from build123d import *

# Parameters (mm, degrees)
SKETCH1_W           = 25
SKETCH1_H           = 7.15
BOSS_EXTRUDE1_DEPTH = 12
BOSS_EXTRUDE2_DEPTH = 3
CUT_EXTRUDE1_DEPTH  = 21
SKETCH4_R           = 9
CUT_EXTRUDE2_DEPTH  = 10
CHAMFER1_SIZE       = 5
CHAMFER1_SIZE2      = 20
CHAMFER2_SIZE       = 5
SKETCH6_R           = 1.05
CUT_EXTRUDE3_DEPTH  = 10
CUT_EXTRUDE4_DEPTH  = 4.5
FILLET1_R           = 3
FILLET2_R           = 1.5


with BuildPart() as part:
    # Sketch1 → Boss-Extrude1 (new body)
    with BuildSketch(Plane.XY):
        with Locations((12.5, 3.575)):
            Rectangle(SKETCH1_W, SKETCH1_H)
    extrude(amount=BOSS_EXTRUDE1_DEPTH)

    # Sketch2 → Boss-Extrude2 (add)
    with BuildSketch(Plane(origin=(0, 7.15, 0), x_dir=(1, 0, 0), z_dir=(0, 1, 0))):
        with BuildLine():
            Line((15, -12), (15, -6))
            Line((15, -6), (15, 0))
            Line((15, 0), (-5.804949202, 4.737516245))
            ThreePointArc((-5.804949202, 4.737516245), (-19.262380692, -6), (-5.804949202, -16.737516245))
            Line((-5.804949202, -16.737516245), (15, -12))
        make_face()
    extrude(amount=-BOSS_EXTRUDE2_DEPTH)

    # Sketch3 → Cut-Extrude1 (cut)
    with BuildSketch(Plane.XZ.offset(-4.15)):
        Polygon((2.25, 6), (2.25, 12), (0, 12), (0, 0), (2.25, 0), align=None)
    extrude(amount=CUT_EXTRUDE1_DEPTH, mode=Mode.SUBTRACT)

    # Sketch4 → Cut-Extrude2 (cut)
    with BuildSketch(Plane.XZ.offset(-4.15)):
        with Locations(Location((-8.25, 6, 0), (0, 0, 270))):
            Circle(SKETCH4_R)
    extrude(amount=-CUT_EXTRUDE2_DEPTH, mode=Mode.SUBTRACT)

    # Chamfer1
    chamfer1_edges = [part.edges().sort_by_distance(p)[0] for p in [
        (25, 7.15, 6),
    ]]
    chamfer1_side = [part.faces().sort_by_distance(p)[0] for p in [
        (25, 3.575, 6),
    ]]
    chamfer(chamfer1_edges, length=CHAMFER1_SIZE, length2=CHAMFER1_SIZE2, reference=chamfer1_side[0])

    # Chamfer2
    chamfer2_edges = [part.edges().sort_by_distance(p)[0] for p in [
        (25, 1.075, 0),
        (25, 1.075, 12),
    ]]
    chamfer(chamfer2_edges, length=CHAMFER2_SIZE)

    # Sketch6 → Cut-Extrude3 (cut)
    with BuildSketch(Plane(origin=(0, 7.15, 0), x_dir=(1, 0, 0), z_dir=(0, 1, 0))):
        with Locations(Location((7.829893366, -6, 0), (0, 0, 180))):
            Circle(SKETCH6_R)
        with Locations(Location((17.829893366, -6, 0), (0, 0, 180))):
            Circle(SKETCH6_R)
    extrude(amount=-CUT_EXTRUDE3_DEPTH, mode=Mode.SUBTRACT)

    # Sketch7 → Cut-Extrude4 (cut)
    with BuildSketch(Plane(origin=(0, 7.15, 0), x_dir=(1, 0, 0), z_dir=(0, 1, 0))):
        with BuildLine():
            Line((7.829893366, -2), (17.829893366, -2))
            ThreePointArc((17.829893366, -2), (21.829893366, -6), (17.829893366, -10))
            Line((17.829893366, -10), (7.829893366, -10))
            ThreePointArc((7.829893366, -10), (3.829893366, -6), (7.829893366, -2))
        make_face()
    extrude(amount=-CUT_EXTRUDE4_DEPTH, mode=Mode.SUBTRACT)

    # Fillet1
    fillet1_edges = [part.edges().sort_by_distance(p)[0] for p in [
        (2.25, 2.075, 0),
        (2.25, 2.075, 12),
    ]]
    fillet(fillet1_edges, radius=FILLET1_R)

    # Fillet2
    fillet2_edges = [part.edges().sort_by_distance(p)[0] for p in [
        (10.125, 4.15, 0),
        (3.128679656, 4.15, 0.878679656),
        (2.25, 4.15, 6),
        (3.128679656, 4.15, 11.121320344),
        (10.125, 4.15, 12),
    ]]
    fillet(fillet2_edges, radius=FILLET2_R)


solid = part.part
Model file for the job. Use its own axes, mm. A direction names the side the tool comes from. Round coordinates to 2 decimals unless told otherwise and drop trailing zeros. Order: outer loops, then holes, each group sorted by start corner. A loop starts at its lowest first (then second) coordinate and runs counter-clockwise, first axis right, second up.
(1) Pull direction X, two halves, no side cores. Call faces 1 (the face through (6.83, 1.34, 6.32)), 2 (the face through (13, 2, 12)), 3 (the face through (13.472, 5.032, 1.67)): released by +X, released by -X, zero draft, split by the parting line, or undercut.
(2) Band-saw the part on B-B (y = 1). List the corners of the cut face in (x, z), then the cut area to 3 significant figures.
(3) Band-saw the part on C-C (z = 5.5). Give the number of separate pieces and of enclosed holes in the cut face, then the cut area to 3 significant figures.
(4) 3-axis set-ups, long thin cutter, end or side, ignore diameter. For faces 4 (the face through (3.15, 1.31, 11.14)), 5 (the face through (3.15, 1.31, 0.86)), 6 (the face through (3.83, 4.93, 6.09)): which of +Z, -Z, +X, -X, +Y, -Y reach the whole face in a straight line?
(5) Pin check, flat tips, straight feed: pin 1 (3 mm diameter, centred on x = 14.5, y = 4, fed in from +Z); pin 2 (11 mm diameter, centred on x = -4.5, z = 6.5, fed in from -Y); pin 3 (3 mm diameter, centred on x = 11.5, y = 5, fed in from -Z); pin 4 (1.9 mm diameter, centred on x = 7.83, z = 6, fed in from -Y). Stop position of each tip, or through.
(6) Band-saw the part on D-D (x = 16). List the corners of the cut face in (y, z).
(7) Band-saw the part on A-A (x = -8.25). List the corners of the cut face in (y, z).
(8) Drill centre lines: line 1 (X direction, y = 6.15, z = 6); line 2 (Y direction, x = -5, z = 14.5); line 3 (Y direction, x = 14.5, z = 4). Where is each one in solid material? Low to high.
Verdict:
1. face 1: undercut
1. face 2: zero draft
1. face 3: released by +X
2. outline: (2.25, 3) arc R3 ccw to (5.25, 0) - (20, 0) - (25, 5) - (25, 7) - (20, 12) - (5.25, 12) arc R3 ccw to (2.25, 9) - close; hole circle Ø2.1 at (7.83, 6); hole circle Ø2.1 at (17.83, 6)
2. area: 237 mm2
3. separate pieces: 4
3. enclosed holes: 0
3. area: 68.5 mm2
4. face 4: +Z, -X, -Y
4. face 5: -Z, -X, -Y
4. face 6: +Y
5. pin 1: stops at z = 12.46
5. pin 2: stops at y = 4.13
5. pin 3: stops at z = -1.14
5. pin 4: passes through
6. outline: (0, 0) - (4.4, 0) - (4.4, 2) - (2.65, 2) - (2.65, 10) - (4.4, 10) - (4.4, 12) - (0, 12) - close
7. outline: (4.15, -5.01) - (7.15, -5.01) - (7.15, -3) - (4.15, -3) - close; (4.15, 15) - (7.15, 15) - (7.15, 17.01) - (4.15, 17.01) - close
8. line 1: x = -19.26 to -17.25, 0.75 to 3.83
8. line 2: y = 4.15 to 7.15
8. line 3: y = 0 to 2.65
